The model under review builds one solid part; all positions refer to its coordinate system, in mm. A direction names the side the tool comes from. Coordinates: 2 decimals unless noted, no trailing zeros. Loops run counter-clockwise (first coordinate to the right, second up) from the corner with the lowest first, then second, coordinate; pieces in that order, holes last. Notation, with made-up numbers: (-31.75, 68) - (-14.75, 68) arc R24 cw to (-14.75, 96) - close; hole circle Ø5 at (46.25, 23.25). An arc over 180 degrees is marked (long way). One line per item, written item: value. Start each with the question number.
1. Insertion check: P1, Ø4, axis at x = -25.5, y = -4.5, coming from the +Z side; P2, Ø2, axis at x = -14.5, z = 12, coming from the -Y side; P3, Ø12, axis at y = -27, z = 10.5, coming from the -X side. Each pin has a flat end and moves straight along its axis. Give the tip position at first contact, or say it passes through.
2. We need section C-C, the plane y = 33.5. Give the boundary of the cut face in (x, z), then the cut area to 3 significant figures.
3. We need section D-D, the plane x = 21. Give the boundary of the cut face in (y, z).
4. For faces 4 (the face through (40, 0, 5)), 5 (the face through (-31.2, 32.6, 12.4)), list the 3-axis set-ups (+Z, -Z, +X, -X, +Y, -Y) from which the entire face can be reached by the end or side of a thin tool; tool diameter is ignored.
5. To check wall thickness, follow line 1 (Y direction, x = -30, z = 14.75); line 2 (Y direction, x = 30, z = 9.75); line 3 (Y direction, x = 7.5, z = 8.5). State the ranges of each line that lie inside material, in increasing order.
6. We need section B-B, the plane z = 7.75. Count the separate pieces of the cut face and the enclosed holes in it, then the cut area to 3 significant figures.
7. Mouldability with a two-part tool opening along Y and no side actions: class faces 1 (the face through (37.719, 41.094, 4.93)), 2 (the face through (31, 35, 20)), 3 (the face through (0, 38.5, 7)) as +Y half, -Y half, draft (parallel to the pull), parting line (faces both ways), or undercut.
8. We need section A-A, the plane z = 12.5. Give the boundary of the cut face in (x, y), then the cut area to 3 significant figures.
from build123d import *

# Parameters (mm, degrees)
F1_DEPTH = 10
F0_R     = 3
F0_R_2   = 1.5
F2_DEPTH = 5
F3_DEPTH = 20


with BuildPart() as f1:
    # F0 (on Top) → F1 (new body)
    with BuildSketch(Plane.XY):
        with BuildLine():
            ThreePointArc((40, 35.5), (37.656854, 41.156854), (32, 43.5))
            Line((32, 43.5), (-32, 43.5))
            ThreePointArc((-32, 43.5), (-37.656854, 41.156854), (-40, 35.5))
            Line((-40, 35.5), (-40, -35.5))
            ThreePointArc((-40, -35.5), (-37.656854, -41.156854), (-32, -43.5))
            Line((-32, -43.5), (32, -43.5))
            ThreePointArc((32, -43.5), (37.656854, -41.156854), (40, -35.5))
            Line((40, -35.5), (40, 35.5))
        make_face()
        with BuildLine():
            Line((-32, 38.5), (32, 38.5))
            ThreePointArc((32, 38.5), (34.12132, 37.62132), (35, 35.5))
            Line((35, 35.5), (35, -35.5))
            ThreePointArc((35, -35.5), (34.12132, -37.62132), (32, -38.5))
            Line((32, -38.5), (-32, -38.5))
            ThreePointArc((-32, -38.5), (-34.12132, -37.62132), (-35, -35.5))
            Line((-35, -35.5), (-35, 35.5))
            ThreePointArc((-35, 35.5), (-34.12132, 37.62132), (-32, 38.5))
        make_face(mode=Mode.SUBTRACT)
    extrude(amount=F1_DEPTH)

    # F0 (on Top) → F2 (join)
    with BuildSketch(Plane.XY):
        with BuildLine():
            ThreePointArc((35, 35.5), (34.12132, 37.62132), (32, 38.5))
            Line((32, 38.5), (-32, 38.5))
            ThreePointArc((-32, 38.5), (-34.12132, 37.62132), (-35, 35.5))
            Line((-35, 35.5), (-35, -35.5))
            ThreePointArc((-35, -35.5), (-34.12132, -37.62132), (-32, -38.5))
            Line((-32, -38.5), (32, -38.5))
            ThreePointArc((32, -38.5), (34.12132, -37.62132), (35, -35.5))
            Line((35, -35.5), (35, 35.5))
        make_face()
        with Locations((-30, -33.5)):
            Circle(F0_R, mode=Mode.SUBTRACT)
        with Locations((30, -33.5)):
            Circle(F0_R, mode=Mode.SUBTRACT)
        with Locations((-30, 33.5)):
            Circle(F0_R, mode=Mode.SUBTRACT)
        with Locations((30, 33.5)):
            Circle(F0_R, mode=Mode.SUBTRACT)
        with Locations((-30, -33.5)):
            Circle(F0_R_2)
        with Locations((30, -33.5)):
            Circle(F0_R_2)
        with Locations((30, 33.5)):
            Circle(F0_R_2)
        with Locations((-30, 33.5)):
            Circle(F0_R_2)
    extrude(amount=F2_DEPTH)

    # F0 (on Top) → F3 (join)
    with BuildSketch(Plane.XY):
        with Locations((-30, 33.5)):
            Circle(F0_R)
        with Locations((-30, 33.5)):
            Circle(F0_R_2, mode=Mode.SUBTRACT)
        with Locations((30, 33.5)):
            Circle(F0_R)
        with Locations((30, 33.5)):
            Circle(F0_R_2, mode=Mode.SUBTRACT)
        with Locations((30, -33.5)):
            Circle(F0_R)
        with Locations((30, -33.5)):
            Circle(F0_R_2, mode=Mode.SUBTRACT)
        with Locations((-30, -33.5)):
            Circle(F0_R)
        with Locations((-30, -33.5)):
            Circle(F0_R_2, mode=Mode.SUBTRACT)
    extrude(amount=F3_DEPTH)


solid = f1.part
Findings below:
1. P1: z = 5
1. P2: through
1. P3: x = -40
2. outline: (-40, 0) - (40, 0) - (40, 10) - (35, 10) - (35, 5) - (33, 5) - (33, 20) - (31.5, 20) - (31.5, 5) - (28.5, 5) - (28.5, 20) - (27, 20) - (27, 5) - (-27, 5) - (-27, 20) - (-28.5, 20) - (-28.5, 5) - (-31.5, 5) - (-31.5, 20) - (-33, 20) - (-33, 5) - (-35, 5) - (-35, 10) - (-40, 10) - close
2. area: 540 mm2
3. outline: (-43.5, 0) - (43.5, 0) - (43.5, 10) - (38.5, 10) - (38.5, 5) - (-38.5, 5) - (-38.5, 10) - (-43.5, 10) - close
4. face 4: +Z, -Z, +X, +Y, -Y
4. face 5: +Z
5. line 1: -36.5 to -35, -32 to -30.5, 30.5 to 32, 35 to 36.5
5. line 2: -43.5 to -38.5, -36.5 to -35, -32 to -30.5, 30.5 to 32, 35 to 36.5, 38.5 to 43.5
5. line 3: -43.5 to -38.5, 38.5 to 43.5
6. separate pieces: 5
6. enclosed holes: 5
6. area: 1,610 mm2
7. face 1: +Y half
7. face 2: draft
7. face 3: undercut
8. outline: circle Ø6 at (-30, -33.5); circle Ø6 at (-30, 33.5); circle Ø6 at (30, -33.5); circle Ø6 at (30, 33.5); hole circle Ø3 at (-30, -33.5); hole circle Ø3 at (-30, 33.5); hole circle Ø3 at (30, -33.5); hole circle Ø3 at (30, 33.5)
8. area: 84.8 mm2
